Check sheet for the modelled part. Datum: model origin and axes. Units: mm. A direction names the side the tool comes from. Give positions to 0.01 mm unless a question says otherwise; leave off trailing zeros. Order: outer loops, then holes, each group sorted by start corner. A loop starts at its lowest first (then second) coordinate and runs counter-clockwise, first axis right, second up. Notation, with made-up numbers: M 1.5,5.5 L 22.5,5.5 A32 cw 22.5,34.5 Z; hole C 42,4 d6. An arc over 180 degrees is marked long. Return JSON: item names as keys, results as strings. Group by question number.
from build123d import *

# Parameters (mm, degrees)
SKETCH_R        = 27.5
SKETCH_R_2      = 23.5
PAD_DEPTH       = 5
SKETCH001_R     = 1.5
POCKET_DEPTH    = 10
SKETCH002_R     = 1.5
POCKET001_DEPTH = 1.5


with BuildPart() as part:
    # Sketch → Pad (new body)
    with BuildSketch(Plane.XY):
        Circle(SKETCH_R)
        Circle(SKETCH_R_2, mode=Mode.SUBTRACT)
    extrude(amount=PAD_DEPTH)

    # Sketch001 → Pocket (cut)
    with BuildSketch(Plane(origin=(27.5, 0, 0), x_dir=(1, 0, 0), z_dir=(0, 0, 1))):
        Circle(SKETCH001_R)
    extrude(amount=POCKET_DEPTH, mode=Mode.SUBTRACT)

    # Sketch002 → Pocket001 (cut)
    with BuildSketch(Plane.YZ.offset(27.5)):
        Circle(SKETCH002_R)
    extrude(amount=-POCKET001_DEPTH, mode=Mode.SUBTRACT)


solid = part.part
1) Sectioned sample at B-B on y = -6. Record the boundary of the cut face in (x, z).
2) Release check for a two-part mould opening along X. For faces 3 (the face through (26, 0, 1)), 4 (the face through (20.2, 12.4, 5)), 5 (the face through (22.4, 7.1, 2.5)) record: released by +X, released by -X, zero draft, split by the parting line, or undercut.
3) Sectioned sample at C-C on z = 4.3. Record the boundary of the cut face in (x, y), then the cut area to 3 significant figures.
4) Sectioned sample at A-A on x = 0. Record the boundary of the cut face in (y, z).
5) Tool access check on faces 1 (the face through (26.42, -1.35, 0.65)), 2 (the face through (-27.474, 1.188, 2.465)). Record the directions out of +Z, -Z, +X, -X, +Y, -Y that give a thin tool (end or side, any length) a straight path to the whole face; none if there is none.
6) Material ranges on line 1 along Y through (x, z) = (0, 2.05); line 2 along X through (y, z) = (6, 1.15); line 3 along X through (y, z) = (-1, 4.6), recorded low to high.
7) Depth check by flat-ended pin: P1, Ø1, axis at y = -17, z = 2, coming from the +X side; P2, Ø2, axis at y = -21.5, z = 2, coming from the +X side; P3, Ø3, axis at y = 2, z = 1.5, coming from the -X side. Enter the tip coordinate at first touch or a pass-through.
Reply:
{
 "1": {"outline": "M -26.84,0 L -22.72,0 L -22.72,5 L -26.84,5 Z; M 22.72,0 L 26.84,0 L 26.84,5 L 22.72,5 Z"},
 "2": {"face 3": "released by +X", "face 4": "zero draft", "face 5": "undercut"},
 "3": {"outline": "M 27.46,-1.5 A1.5 cw 27.46,1.5 A27.5 ccw long Z; hole C 0,0 d47", "area": "637 mm^2"},
 "4": {"outline": "M -27.5,0 L -23.5,0 L -23.5,5 L -27.5,5 Z; M 23.5,0 L 27.5,0 L 27.5,5 L 23.5,5 Z"},
 "5": {"face 1": "-Z, +X", "face 2": "+Z, -Z"},
 "6": {"line 1": "-27.5 to -23.5, 23.5 to 27.5", "line 2": "-26.84 to -22.72, 22.72 to 26.84", "line 3": "-27.48 to -23.48, 23.48 to 26.38"},
 "7": {"P1": "x = 22", "P2": "x = 18.33", "P3": "x = -27.5"}
}
